from build123d import *

# Parameters (mm, degrees)
F0_W      = 118.7055855989
F0_H      = 68.5793161392
F1_DEPTH  = 50.8
F2_R      = 5.08
F2_R_2    = 5.0799985524
F3_DEPTH  = 101.6
F4_DEPTH  = 12.446
F5_DEPTH  = 82.042
F7_DEPTH  = 187.96
F9_DEPTH  = 14.986
F10_W     = 14.8076536134
F10_H     = 8.8449797213
F11_DEPTH = 191.262


with BuildPart() as f1:
    # F0 (on Top) → F1 (new body)
    with BuildSketch(Plane.XY):
        Rectangle(F0_W, F0_H)
    extrude(amount=F1_DEPTH)

    # F2 (on face) → F3 (cut)
    with BuildSketch(Plane.YZ.offset(59.3527927995)):
        with Locations((-17.0466899602, 12.81891503)):
            Circle(F2_R)
        with Locations((21.4545419486, 12.81891503)):
            Circle(F2_R_2)
        with Locations((21.4545419486, 37.8581796117)):
            Circle(F2_R)
        with Locations((-17.0466899602, 37.8581796117)):
            Circle(F2_R)
    extrude(amount=-F3_DEPTH, mode=Mode.SUBTRACT)

    # F4 (add): a face of the model
    f4_faces = [f1.faces().sort_by_distance(p)[0] for p in [
        (0, -34.2896580696, 25.4),
    ]]
    extrude(f4_faces, amount=F4_DEPTH)

    # F5 (cut): faces of the model
    f5_faces = [f1.faces().sort_by_distance(p)[0] for p in [
        (-42.2472072005, -17.0466899602, 37.8581796117),
        (-42.2472072005, 21.4545419486, 12.81891503),
        (-42.2472072005, -17.0466899602, 12.81891503),
        (-42.2472072005, 21.4545419486, 37.8581796117),
    ]]
    extrude(f5_faces, amount=-F5_DEPTH, mode=Mode.SUBTRACT)

    # F6 (on face) → F7 (cut)
    with BuildSketch(Plane.XZ.offset(46.7356580696)):
        Polygon((59.3527927995, 50.8), (0, 50.8), (59.3527927995, 0), align=None)
    extrude(amount=-F7_DEPTH, mode=Mode.SUBTRACT)

    # F8 (on face) → F9 (cut)
    with BuildSketch(Plane.XZ.offset(46.7356580696)):
        Polygon((59.3527927995, 0), (13.7639556508, 39.0194431959), (13.7639556508, 0), align=None)
    extrude(amount=-F9_DEPTH, mode=Mode.SUBTRACT)

    # F10 (on face) → F11 (cut)
    with BuildSketch(Plane(origin=(-59.3527927995, 0, 0), x_dir=(0, -1, 0), z_dir=(-1, 0, 0))):
        with Locations((0, 46.3775101393)):
            Rectangle(F10_W, F10_H)
        with Locations((0, 55.2224898607)):
            Rectangle(F10_W, F10_H)
    extrude(amount=-F11_DEPTH, mode=Mode.SUBTRACT)


solid = f1.part
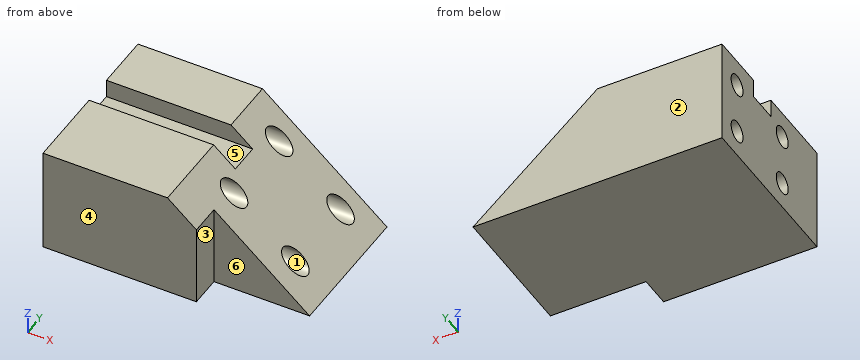
The listing builds one solid part. Answer for the finished solid, in the listing's coordinates (mm). Face numbers are marked on the shaded views. A direction names the side the tool comes from. Round coordinates to 2 decimals unless told otherwise and drop trailing zeros. Write each loop counter-clockwise with the first axis right and the second up, starting at its lowest first coordinate (ties: lowest second). Pieces come first, ordered by that corner, then holes. Notation, with made-up numbers: M -16.5,88 L 24.5,88 A23 cw 24.5,112 Z; hole C 10,-23 d3. An arc over 180 degrees is marked long. Write each question's results on one line, items separated by ' | '. Start each with the question number.
(1) For the marked faces 4, 5 and 6, determine the directions among +Z, -Z, +X, -X, +Y, -Y from which every point of the face is accessible in a straight line to the end or side of a thin tool.
(2) The part is cut by section C-C, the plane x = -17. Write down the section's boundary in (y, z).
(3) Find the intervals of material crossed by line 1 (Z direction, x = -42, y = -13); line 2 (Y direction, x = -24.5, z = 45); line 3 (Z direction, x = -36.5, y = 19.5), in increasing order.
(4) The part is cut by section A-A, the plane z = 9. Write down the section's boundary in (x, y), and give its area (3 significant figures).
(5) The part is cut by section B-B, the plane y = -15.5. Write down the section's boundary in (x, z).
(6) Each of these flat-tipped pins is pushed along its axis until it touches: P1, Ø1, axis at y = -32.5, z = 13, coming from the +X side; P2, Ø16.5, axis at y = -17.05, z = 12.82, coming from the +X side; P3, Ø6, axis at x = 33, z = 17.5, coming from the -Y side. Where does it stop, or does it pass through?
(7) The part is cut by section D-D, the plane y = -33.5. Write down the section's boundary in (x, z).
(8) Determine the mould class of the marked faces 1, 2 and 3 for opening direction Y: +Y half, -Y half, draft (parallel to the pull), parting line (faces both ways), or undercut.
Worked answers:
1) face 4: +Z, -Z, +X, -X, -Y | face 5: +Z, +X, -X | face 6: +Z, -Z, +X, -Y
2) outline: M -46.74,0 L 34.29,0 L 34.29,50.8 L 7.4,50.8 L 7.4,41.96 L -7.4,41.96 L -7.4,50.8 L -46.74,50.8 Z; hole C -17.05,12.82 d10.16; hole C -17.05,37.86 d10.16; hole C 21.45,12.82 d10.16; hole C 21.45,37.86 d10.16
3) line 1: z = 0 to 9.75, 15.89 to 34.79, 40.93 to 50.8 | line 2: y = -46.74 to -7.4, 7.4 to 34.29 | line 3: z = 0 to 8.13, 17.51 to 33.17, 42.55 to 50.8
4) outline: M -59.35,-46.74 L 13.76,-46.74 L 13.76,-31.75 L 48.84,-31.75 L 48.84,-20.4 L -59.35,-20.4 Z; M -59.35,-13.7 L 48.84,-13.7 L 48.84,18.1 L -59.35,18.1 Z; M -59.35,24.8 L 48.84,24.8 L 48.84,34.29 L -59.35,34.29 Z | area: 6,790 mm²
5) outline: M -59.35,0 L 59.35,0 L 50.03,7.98 L -59.35,7.98 Z; M -59.35,17.66 L 38.72,17.66 L 20.77,33.02 L -59.35,33.02 Z; M -59.35,42.7 L 9.47,42.7 L 0,50.8 L -59.35,50.8 Z
6) P1: stops at x = 13.76 | P2: stops at x = 54.01 | P3: stops at y = -31.75
7) outline: M -59.35,0 L 13.76,0 L 13.76,39.02 L 0,50.8 L -59.35,50.8 Z
8) face 1: undercut | face 2: +Y half | face 3: draft
